from build123d import *

# Parameters (mm, degrees)
SKETCH_1_W          = 6
SKETCH_1_H          = 6
EXTRUDE_1_DEPTH     = 4.5
FILLET_1_R          = 1.5
FILLET_3_R          = 0.5
SKETCH_2_W          = 7
SKETCH_2_H          = 7
EXTRUDE_2_DEPTH     = 4.7
SKETCH_5_W          = 7
SKETCH_5_H          = 7
CUT_EXTRUDE_1_DEPTH = 1.7


with BuildPart() as part:
    # 草图1 → 凸台-拉伸1 (new body)
    with BuildSketch(Plane(origin=(0, 0, 0), x_dir=(1, 0, 0), z_dir=(0, 1, 0))):
        Rectangle(SKETCH_1_W, SKETCH_1_H)
    extrude(amount=EXTRUDE_1_DEPTH)

    # 圆角1
    fillet_1_edges = [part.edges().sort_by_distance(p)[0] for p in [
        (3, 2.25, 3),
        (-3, 2.25, 3),
        (-3, 2.25, -3),
        (3, 2.25, -3),
    ]]
    fillet(fillet_1_edges, radius=FILLET_1_R)

    # 圆角3
    fillet_3_edges = [part.edges().sort_by_distance(p)[0] for p in [
        (-3, 4.5, 0),
        (0, 4.5, -3),
        (3, 4.5, 0),
        (0, 4.5, 3),
        (-2.560660172, 4.5, 2.560660172),
        (2.560660172, 4.5, 2.560660172),
        (2.560660172, 4.5, -2.560660172),
        (-2.560660172, 4.5, -2.560660172),
    ]]
    fillet(fillet_3_edges, radius=FILLET_3_R)

    # 草图2 → 凸台-拉伸2 (add)
    with BuildSketch(Plane.XZ):
        Rectangle(SKETCH_2_W, SKETCH_2_H)
    extrude(amount=EXTRUDE_2_DEPTH)

    # 切除-放样1: read off the stored shape, not the designer's step
    # 切除-放样1: loft between two sections, ruled curve by curve
    loft_1_from = [
        Edge.make_bspline([(1.999712209, -4.7, -0.033927573), (1.931857063, -4.7, -4.033351992), (-2.067567356, -4.7, -3.965496845), (-1.999712209, -4.7, 0.033927573), (-1.931857063, -4.7, 4.033351992), (2.067567356, -4.7, 3.965496845), (1.999712209, -4.7, -0.033927573)], [0, 0, 0, 0, 0.5, 0.5, 0.5, 1, 1, 1, 1], 3, [1, 0.333333333, 0.333333333, 1, 0.333333333, 0.333333333, 1]),
    ]
    loft_1_to = [
        Edge.make_bspline([(1.873751703, 0.3, 0.314729335), (2.503210373, 0.3, -3.432774072), (-1.244293034, 0.3, -4.062232741), (-1.873751703, 0.3, -0.314729335), (-2.503210373, 0.3, 3.432774072), (1.244293034, 0.3, 4.062232741), (1.873751703, 0.3, 0.314729335)], [0, 0, 0, 0, 0.5, 0.5, 0.5, 1, 1, 1, 1], 3, [1, 0.333333333, 0.333333333, 1, 0.333333333, 0.333333333, 1]),
    ]
    loft_1 = Solid(Shell([*[Face.make_surface_from_curves(loft_1_from[k], loft_1_to[k]) for k in range(1)], Face(Wire(loft_1_from)), Face(Wire(loft_1_to))]))
    add(loft_1, mode=Mode.SUBTRACT)

    # 草图5 → 切除-拉伸1 (cut)
    with BuildSketch(Plane.XZ.offset(4.7)):
        Rectangle(SKETCH_5_W, SKETCH_5_H)
    extrude(amount=-CUT_EXTRUDE_1_DEPTH, mode=Mode.SUBTRACT)


solid = part.part
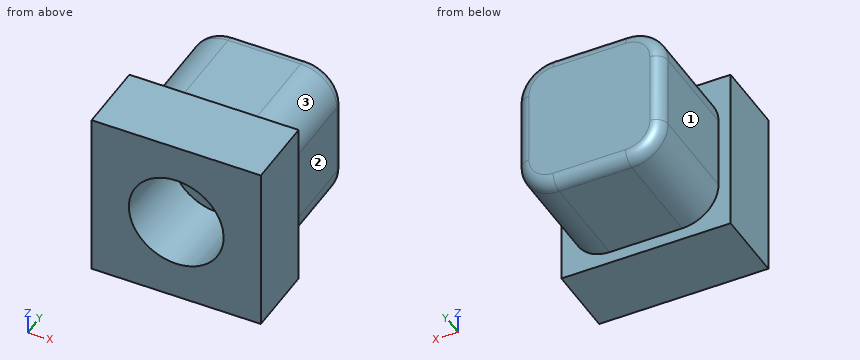
CAD build for the part. Positions are in the model's coordinates, mm. Face numbers are marked on the shaded views. A direction names the side the tool comes from. Round coordinates to 2 decimals unless told otherwise and drop trailing zeros. Order: outer loops, then holes, each group sorted by start corner. A loop starts at its lowest first (then second) coordinate and runs counter-clockwise, first axis right, second up. Notation, with made-up numbers: (16, 58) -> (59, 58) arc R24 cw to (59, 95) -> close; hole circle Ø3 at (42.5, -28). An arc over 180 degrees is marked (long way). Write each question's results on one line, items separated by ' | '.
1. Wall check: line 1 along Y through (x, z) = (-0.25, -1.25); line 2 along X through (y, z) = (-2, -0.25); line 3 along Z through (x, y) = (0.75, 2.75). Give the ranges that are in metal, low to high. Write a range as [from, to].
Findings below:
line 1: y = [0.3, 4.5] | line 2: x = [-3.5, -1.92], [1.92, 3.5] | line 3: z = [-3, 3]
2. Flat gauge pins, fed straight in: P1, Ø1.5, axis at y = 3, z = 0, coming from the -X side; P2, Ø1.5, axis at y = 2, z = 0.5, coming from the +X side; P3, Ø2.5, axis at x = 0.5, y = 2.5, coming from the +Z side. Where does each tip first touch, or does it go through?
Findings below:
P1: stops at x = -3 | P2: stops at x = 3 | P3: stops at z = 3
3. 3-axis set-ups, long thin cutter, end or side, ignore diameter. For the marked faces 1, 2 and 3: which of +Z, -Z, +X, -X, +Y, -Y reach the whole face in a straight line?
Findings below:
face 1: +Z, -Z, -X, +Y | face 2: +Z, -Z, +X, +Y | face 3: +Z, +X, +Y
4. Cut at A-A (y = 2). Give the cut face in (x, z).
Findings below:
outline: (-3, -1.5) arc R1.5 ccw to (-1.5, -3) -> (1.5, -3) arc R1.5 ccw to (3, -1.5) -> (3, 1.5) arc R1.5 ccw to (1.5, 3) -> (-1.5, 3) arc R1.5 ccw to (-3, 1.5) -> close
5. Cut at B-B (z = 3.25). Give the cut face in (x, y), plus the area to 3 significant figures.
Findings below:
outline: (-3.5, -3) -> (3.5, -3) -> (3.5, 0) -> (-3.5, 0) -> close | area: 21.0 mm²
